```python
from build123d import *

# Parameters (mm, degrees)
SKETCH1_W             = 50.8
SKETCH1_H             = 76.2
BOSS_EXTRUDE1_DEPTH   = 1150
SKETCH2_W             = 46.8
SKETCH2_H             = 72.2
CUT_EXTRUDE1_DEPTH    = 1151.911278075
FILLET2_R             = 2
CROQUIS1_R            = 2.5
CORTAR_EXTRUIR1_DEPTH = 5
MATRIZL1_COUNT        = 4
MATRIZL1_PITCH        = 357.9333
CROQUIS2_R            = 2.5
CORTAR_EXTRUIR2_DEPTH = 10
CROQUIS3_R            = 2.5
CORTAR_EXTRUIR3_DEPTH = 10
CROQUIS4_R            = 2.5
CORTAR_EXTRUIR4_DEPTH = 10
MATRIZL2_COUNT        = 18
MATRIZL2_PITCH        = 60
CROQUIS5_R            = 2.5
CORTAR_EXTRUIR5_DEPTH = 10


with BuildPart() as part:
    # Sketch1 → Boss-Extrude1 (new body)
    with BuildSketch(Plane(origin=(0, 0, 0), x_dir=(0, 0, -1), z_dir=(1, 0, 0))):
        Rectangle(SKETCH1_W, SKETCH1_H)
    extrude(amount=-BOSS_EXTRUDE1_DEPTH)

    # Sketch2 → Cut-Extrude1 (cut, through all)
    with BuildSketch(Plane(origin=(0, 0, 0), x_dir=(0, 0, -1), z_dir=(1, 0, 0))):
        Rectangle(SKETCH2_W, SKETCH2_H)
    extrude(amount=-CUT_EXTRUDE1_DEPTH, mode=Mode.SUBTRACT)

    # Fillet2
    fillet2_edges = [part.edges().sort_by_distance(p)[0] for p in [
        (-575, -36.1, 23.4),
        (-575, 36.1, 23.4),
        (-575, 36.1, -23.4),
        (-575, -36.1, -23.4),
        (-575, 38.1, 25.4),
        (-575, 38.1, -25.4),
        (-575, -38.1, -25.4),
        (-575, -38.1, 25.4),
    ]]
    fillet(fillet2_edges, radius=FILLET2_R)

    # Croquis1 → Cortar-Extruir1 (cut)
    with BuildSketch(Plane.XZ.offset(38.1)):
        with Locations(Location((-38.1, 0, 0), (0, 0, 270))):
            Circle(CROQUIS1_R)
        with Locations(Location((-61.2, 15.4, 0), (0, 0, 270))):
            Circle(CROQUIS1_R)
        with Locations(Location((-15, 15.4, 0), (0, 0, 270))):
            Circle(CROQUIS1_R)
        with Locations(Location((-15, -15.4, 0), (0, 0, 270))):
            Circle(CROQUIS1_R)
        with Locations(Location((-61.2, -15.4, 0), (0, 0, 270))):
            Circle(CROQUIS1_R)
    cortar_extruir1 = extrude(amount=-CORTAR_EXTRUIR1_DEPTH, mode=Mode.SUBTRACT)

    # MatrizL1: Cortar-Extruir1 ×4
    with Locations(*[(-i * MATRIZL1_PITCH, 0, 0) for i in range(1, MATRIZL1_COUNT)]):
        add(cortar_extruir1, mode=Mode.SUBTRACT)

    # Croquis2 → Cortar-Extruir2 (cut)
    with BuildSketch(Plane(origin=(0, 0, -25.4), x_dir=(-1, 0, 0), z_dir=(0, 0, -1))):
        with Locations(Location((1100, 8.1, 0), (0, 0, 90))):
            Circle(CROQUIS2_R)
        with Locations(Location((225, 8.1, 0), (0, 0, 90))):
            Circle(CROQUIS2_R)
        with Locations(Location((75, -18.1, 0), (0, 0, 90))):
            Circle(CROQUIS2_R)
        with Locations(Location((325, -18.1, 0), (0, 0, 90))):
            Circle(CROQUIS2_R)
        with Locations(Location((675, -18.1, 0), (0, 0, 90))):
            Circle(CROQUIS2_R)
        with Locations(Location((1025, -18.1, 0), (0, 0, 90))):
            Circle(CROQUIS2_R)
    extrude(amount=-CORTAR_EXTRUIR2_DEPTH, mode=Mode.SUBTRACT)

    # Croquis3 → Cortar-Extruir3 (cut)
    with BuildSketch(Plane(origin=(0, 38.1, 0), x_dir=(1, 0, 0), z_dir=(0, 1, 0))):
        with Locations(Location((-31, 17.9, 0), (0, 0, 270))):
            Circle(CROQUIS3_R)
        with Locations(Location((-89, 17.9, 0), (0, 0, 270))):
            Circle(CROQUIS3_R)
        with Locations(Location((-152, 17.9, 0), (0, 0, 270))):
            Circle(CROQUIS3_R)
        with Locations(Location((-152, -17.9, 0), (0, 0, 270))):
            Circle(CROQUIS3_R)
        with Locations(Location((-89, -17.9, 0), (0, 0, 270))):
            Circle(CROQUIS3_R)
        with Locations(Location((-31, -17.9, 0), (0, 0, 270))):
            Circle(CROQUIS3_R)
    extrude(amount=-CORTAR_EXTRUIR3_DEPTH, mode=Mode.SUBTRACT)

    # Croquis4 → Cortar-Extruir4 (cut)
    with BuildSketch(Plane(origin=(0, 38.1, 0), x_dir=(1, 0, 0), z_dir=(0, 1, 0))):
        with Locations(Location((-1117, 0, 0), (0, 0, 270))):
            Circle(CROQUIS4_R)
    cortar_extruir4 = extrude(amount=-CORTAR_EXTRUIR4_DEPTH, mode=Mode.SUBTRACT)

    # MatrizL2: Cortar-Extruir4 ×18
    with Locations(*[(i * MATRIZL2_PITCH, 0, 0) for i in range(1, MATRIZL2_COUNT)]):
        add(cortar_extruir4, mode=Mode.SUBTRACT)

    # Croquis5 → Cortar-Extruir5 (cut)
    with BuildSketch(Plane(origin=(0, 38.1, 0), x_dir=(1, 0, 0), z_dir=(0, 1, 0))):
        with Locations(Location((-1121.5, 16.4, 0), (0, 0, 270))):
            Circle(CROQUIS5_R)
        with Locations(Location((-1121.5, -16.4, 0), (0, 0, 270))):
            Circle(CROQUIS5_R)
        with Locations(Location((-1139, 0, 0), (0, 0, 270))):
            Circle(CROQUIS5_R)
    extrude(amount=-CORTAR_EXTRUIR5_DEPTH, mode=Mode.SUBTRACT)


solid = part.part
```
Could you check a few things on this model? Use its own coordinates, in mm. A direction names the side the tool comes from. Round coordinates to 2 decimals unless told otherwise and drop trailing zeros. Loops run counter-clockwise (first coordinate to the right, second up) from the corner with the lowest first, then second, coordinate; pieces in that order, holes last. Notation, with made-up numbers: (80, -8) - (131, -8) arc R17 cw to (131, 21) - close; hole circle Ø6 at (-31.75, 62). An arc over 180 degrees is marked (long way). Use CSV: the item, a comma, the result in double quotes.
Item 1: If we section it at A-A on x = -838: List the corners of the cut face in (y, z) for me, then the cut area to 3 significant figures.
Here are the results:
outline,"(-38.1, -23.4) arc R2 ccw to (-36.1, -25.4) - (36.1, -25.4) arc R2 ccw to (38.1, -23.4) - (38.1, 23.4) arc R2 ccw to (36.1, 25.4) - (-36.1, 25.4) arc R2 ccw to (-38.1, 23.4) - close; hole (-36.1, -21.4) arc R2 ccw to (-34.1, -23.4) - (34.1, -23.4) arc R2 ccw to (36.1, -21.4) - (36.1, 21.4) arc R2 ccw to (34.1, 23.4) - (-34.1, 23.4) arc R2 ccw to (-36.1, 21.4) - close"
area,"492 mm²"
Item 2: Will this pin go through, and if not, where does the flat tip stop? pin 1 (4.5 mm diameter, centred on x = -937, z = 0, fed in from +Y).
Here are the results:
pin 1,"stops at y = -36.1"
Item 3: I need wall thicknesses on L1, parallel to Z at x = -410, y = 15.5; L2, parallel to Y at x = -1084.5, z = -9; L3, parallel to Z at x = -152, y = 37.1. Which ranges of each line are inside material? Lowest first, please. Write a range as [from, to].
Here are the results:
L1,"z = [-25.4, -23.4], [23.4, 25.4]"
L2,"y = [-38.1, -36.1], [36.1, 38.1]"
L3,"z = [-25.13, -20.4], [-15.4, 15.4], [20.4, 25.13]"
Item 4: If we mould it in two halves opening along Z, with no side actions, what happens to faces 1 (the flat face through (-567, -1, -25.4)), 2 (the flat face through (-1150, 0, 25)), 3 (the flat face through (-567, 36.1, 0))? For each: pulls with the +Z half, pulls with the -Z half, needs draft (parallel to the pull), parting line crosses it, or undercut.
Here are the results:
face 1,"pulls with the -Z half"
face 2,"needs draft"
face 3,"undercut"
Item 5: For faces 4 (the flat face through (-567, 0, -23.4)), 5 (the flat face through (0, 0, 25)), which set-ups out of +Z, -Z, +X, -X, +Y, -Y let a thin tool reach every point of the face, with its end or its side?
Here are the results:
face 4,"+X, -X"
face 5,"+Z, -Z, +X, +Y, -Y"
